The listing builds one solid part. Answer for the finished solid, in the listing's coordinates (mm). A direction names the side the tool comes from. Coordinates: 2 decimals unless noted, no trailing zeros. Order: outer loops, then holes, each group sorted by start corner. A loop starts at its lowest first (then second) coordinate and runs counter-clockwise, first axis right, second up. Notation, with made-up numbers: M 86,47.25 L 127,47.25 A31 ccw 127,72.25 Z; hole C 63.5,34 d2. An arc over 180 degrees is marked long. One line per item, written item: value. Start each with the question number.
Q1. The part is cut by section A-A on y = 15. Give the number of separate pieces and of enclosed holes in the cut face, then the cut area to 3 significant figures.
Q2. For faces 1 (the flat face through (-8.35, 54.97, -13.4)), 2 (the flat face through (12.58, 18.67, -5.71)), 3 (the flat face through (-4.95, 53.99, -7.68)), 4 (the flat face through (2, 35, 10)), determine the directions among +Z, -Z, +X, -X, +Y, -Y from which every point of the face is accessible in a straight line to the end or side of a thin tool.
Q3. Straight lines are drawn through the part: line 1 along Y through (x, z) = (10.5, 2); line 2 along X through (y, z) = (29.5, 0) (3 decimals); line 3 along Y through (x, z) = (-2, -3.25). For each, find the intervals that lie inside material, in ascending order. Write a range as [from, to].
Q4. The part is cut by section B-B on y = 62.5. Give the vertices of the cut face in (x, z) (3 decimals).
Q5. Each of these flat-tipped pins is pushed along its axis until it touches: pin 1 Ø5 at (x, y) = (10.5, 55) entering from -Z (3 decimals); pin 2 Ø6.5 at (x, y) = (7, 52.5) entering from -Z (3 decimals); pin 3 Ø5 at (x, z) = (0, 0) entering from +Y; pin 4 Ø6 at (y, z) = (26, -11) entering from -X. Where does it stop, or does it pass through?
Q6. The part is cut by section C-C on y = 43.5. Give the vertices of the cut face in (x, z) (3 decimals), then the cut area to 3 significant figures.
Q7. Determine the mould class of faces 5 (the flat face through (1, 60, -3)), 6 (the flat face through (-7.2, 34.5, 7.1)), 7 (the flat face through (10, 35, -8.175)) for opening direction X: pulls with the +X half, pulls with the -X half, needs draft (parallel to the pull), parting line crosses it, or undercut.
```python
from build123d import *

# Parameters (mm, degrees)
SKETCH1_R           = 2.0788
BOSS_EXTRUDE1_DEPTH = 70
SKETCH2_R           = 2
CUT_EXTRUDE1_DEPTH  = 15
SKETCH3_R           = 2
CUT_EXTRUDE2_DEPTH  = 15
CUT_EXTRUDE3_DEPTH  = 5
CUT_EXTRUDE4_DEPTH  = 5
CUT_EXTRUDE5_START  = -5
CUT_EXTRUDE5_DEPTH  = 5
FILLET1_R           = 2


with BuildPart() as part:
    # Sketch1 → Boss-Extrude1 (new body)
    with BuildSketch(Plane(origin=(0, 0, 0), x_dir=(1, 0, 0), z_dir=(0, 1, 0))):
        with BuildLine():
            Line((-18.495, 5.34), (-9.495, 17.34))
            Line((-9.495, 17.34), (2.725, 8.175))
            Line((2.725, 8.175), (18, 8.175))
            Line((18, 8.175), (18, -6.825))
            Line((18, -6.825), (3, -6.825))
            Line((3, -6.825), (3, -10))
            Line((3, -10), (0, -10))
            ThreePointArc((0, -10), (-3.16227766, -9.486832981), (-6, -8))
            Line((-6, -8), (-8.4, -6.2))
            Line((-8.4, -6.2), (-6.495, -3.66))
            Line((-6.495, -3.66), (-18.495, 5.34))
        make_face()
        with Locations(Location((0, 0, 0), (0, 0, 270))):
            Circle(SKETCH1_R, mode=Mode.SUBTRACT)
    extrude(amount=BOSS_EXTRUDE1_DEPTH)

    # Sketch2 → Cut-Extrude1 (cut)
    with BuildSketch(Plane.XY.offset(6.825)):
        with Locations((10.5, 15)):
            Circle(SKETCH2_R)
        with Locations((10.5, 55)):
            Circle(SKETCH2_R)
    extrude(amount=-CUT_EXTRUDE1_DEPTH, mode=Mode.SUBTRACT)

    # Sketch3 → Cut-Extrude2 (cut)
    with BuildSketch(Plane(origin=(-4.095, 0, 5.46), x_dir=(0.8000000000000002, 0, 0.5999999999999999), z_dir=(-0.5999999999999999, 0, 0.8000000000000003))):
        with Locations((-10.5, 15)):
            Circle(SKETCH3_R)
        with Locations((-10.5, 55)):
            Circle(SKETCH3_R)
    extrude(amount=-CUT_EXTRUDE2_DEPTH, mode=Mode.SUBTRACT)

    # Sketch4 → Cut-Extrude3 (cut)
    with BuildSketch(Plane(origin=(4.905, 0, -6.54), x_dir=(-0.8000000000000002, 0, -0.5999999999999998), z_dir=(0.5999999999999998, 0, -0.8000000000000002))):
        Polygon((10.5, 59.871392896), (6.28125, 57.435696448), (6.28125, 52.564303552), (10.5, 50.128607104), (14.71875, 52.564303552), (14.71875, 57.435696448), align=None)
        Polygon((10.5, 10.128607104), (14.71875, 12.564303552), (14.71875, 17.435696448), (10.5, 19.871392896), (6.28125, 17.435696448), (6.28125, 12.564303552), align=None)
    extrude(amount=-CUT_EXTRUDE3_DEPTH, mode=Mode.SUBTRACT)

    # Sketch5 → Cut-Extrude4 (cut)
    with BuildSketch(Plane(origin=(0, 0, -8.175), x_dir=(-1, 0, 0), z_dir=(0, 0, -1))):
        Polygon((-10.5, 50.128607104), (-6.28125, 52.564303552), (-6.28125, 57.435696448), (-10.5, 59.871392896), (-14.71875, 57.435696448), (-14.71875, 52.564303552), align=None)
        Polygon((-10.5, 10.128607104), (-6.28125, 12.564303552), (-6.28125, 17.435696448), (-10.5, 19.871392896), (-14.71875, 17.435696448), (-14.71875, 12.564303552), align=None)
    extrude(amount=-CUT_EXTRUDE4_DEPTH, mode=Mode.SUBTRACT)

    # Sketch7 → Cut-Extrude5 (cut)
    with BuildSketch(Plane(origin=(0, 70, 0), x_dir=(1, 0, 0), z_dir=(0, 1, 0)).offset(CUT_EXTRUDE5_START)):
        Polygon((-4.773906582, -0.97690802), (-0.83361646, 10.843962345), (2.725, 8.175), (7.173270575, 8.175), (3.232980454, -3.645870365), (-1.540926128, -4.622778385), align=None)
    extrude(amount=-CUT_EXTRUDE5_DEPTH, mode=Mode.SUBTRACT)

    # Fillet1
    fillet1_edges = [part.edges().sort_by_distance(p)[0] for p in [
        (2.725, 30, -8.175),
        (-18.495, 35, -5.34),
        (-9.495, 35, -17.34),
        (2.725, 67.5, -8.175),
        (18, 35, -8.175),
        (18, 35, 6.825),
    ]]
    fillet(fillet1_edges, radius=FILLET1_R)


solid = part.part
```
Output:
1. separate pieces: 3
1. enclosed holes: 1
1. area: 388 mm^2
2. face 1: +X
2. face 2: -Z
2. face 3: none
2. face 4: +Z, +X, -X, +Y, -Y
3. line 1: y = [0, 13], [17, 53], [57, 70]
3. line 2: x = [-11.375, -2.079], [2.079, 18]
3. line 3: y = [0, 60], [65, 70]
4. outline: M -17.295,-6.94 L -10.695,-15.74 A2 ccw -7.895,-16.14 L -0.834,-10.844 L -4.774,0.977 L -1.541,4.623 L 3.233,3.646 L 7.173,-8.175 L 16,-8.175 A2 ccw 18,-6.175 L 18,4.825 A2 ccw 16,6.825 L 3,6.825 L 3,10 L 0,10 A10 ccw -6,8 L -8.4,6.2 L -6.495,3.66 L -16.895,-4.14 A2 ccw Z
5. pin 1: stops at z = -3.175
5. pin 2: stops at z = -8.175
5. pin 3: stops at y = 70
5. pin 4: stops at x = -16.5
6. outline: M -17.295,-6.94 L -10.695,-15.74 A2 ccw -7.895,-16.14 L 2.192,-8.575 A2 cw 3.392,-8.175 L 16,-8.175 A2 ccw 18,-6.175 L 18,4.825 A2 ccw 16,6.825 L 3,6.825 L 3,10 L 0,10 A10 ccw -6,8 L -8.4,6.2 L -6.495,3.66 L -16.895,-4.14 A2 ccw Z; hole C 0,0 d4.158
6. area: 552 mm^2
7. face 5: undercut
7. face 6: pulls with the -X half
7. face 7: needs draft
